The model under review builds one solid part; all positions refer to its coordinate system, in mm. Face numbers are marked on the shaded views. Coordinates: 2 decimals unless noted, no trailing zeros. Loops run counter-clockwise (first coordinate to the right, second up) from the corner with the lowest first, then second, coordinate; pieces in that order, holes last. Notation, with made-up numbers: M 0,64 L 28,64 A34 cw 28,102 Z; hole C -21,32 d11. An arc over 180 degrees is marked long. Use CSV: the item, a comma, the result in double quotes. Start each with the question number.
from build123d import *

# Parameters (mm, degrees)
SKETCH_1_W          = 40
SKETCH_1_H          = 40
EXTRUDE_1_DEPTH     = 60
SKETCH_7_R          = 2.5
CUT_EXTRUDE_1_DEPTH = 10
SKETCH_8_R          = 2.5
CUT_EXTRUDE_2_DEPTH = 10
SKETCH_10_R         = 12.5
CUT_EXTRUDE_3_DEPTH = 40


with BuildPart() as part:
    # 草图1 → 凸台-拉伸1 (new body)
    with BuildSketch(Plane.XY):
        Rectangle(SKETCH_1_W, SKETCH_1_H)
    extrude(amount=EXTRUDE_1_DEPTH)

    # 草图7 → 切除-拉伸1 (cut)
    with BuildSketch(Plane.XZ.offset(20)):
        with Locations(Location((0, 13, 0), (0, 0, 270))):
            Circle(SKETCH_7_R)
    cut_extrude_1 = extrude(amount=-CUT_EXTRUDE_1_DEPTH, mode=Mode.SUBTRACT)

    # 草图8 → 切除-拉伸2 (cut)
    with BuildSketch(Plane(origin=(20, 0, 0), x_dir=(0, 0, -1), z_dir=(1, 0, 0))):
        with Locations((-13, 0)):
            Circle(SKETCH_8_R)
    cut_extrude_2 = extrude(amount=-CUT_EXTRUDE_2_DEPTH, mode=Mode.SUBTRACT)

    # 镜向1: 切除-拉伸1 across plane
    add(cut_extrude_1.mirror(Plane.ZX), mode=Mode.SUBTRACT)

    # 镜向2: 切除-拉伸2 across plane
    add(cut_extrude_2.mirror(Plane(origin=(0, 0, 0), x_dir=(0, 0, 1), z_dir=(1, 0, 0))), mode=Mode.SUBTRACT)

    # 草图10 → 切除-拉伸3 (cut)
    with BuildSketch(Plane.XY.offset(60)):
        Circle(SKETCH_10_R)
    extrude(amount=-CUT_EXTRUDE_3_DEPTH, mode=Mode.SUBTRACT)


solid = part.part
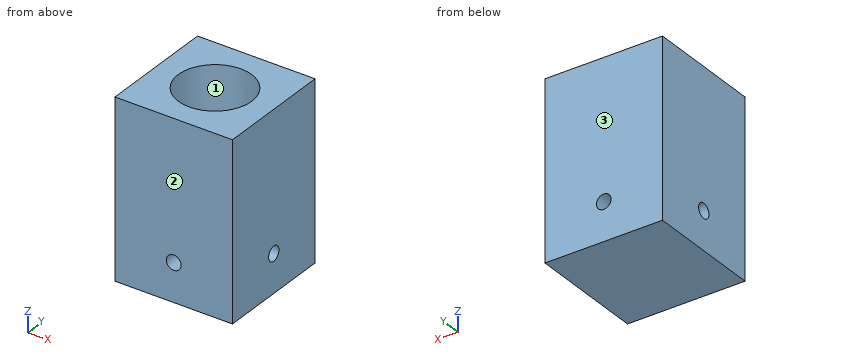
1. Add section B-B (x = 0). Write out the cut boundary in (y, z), plus the area to 3 significant figures.
2. Add section D-D (y = 9). Write out the cut boundary in (x, z), plus the area to 3 significant figures.
3. Add section C-C (z = 28). Write out the cut boundary in (x, y).
4. Add section A-A (z = 11.5). Write out the cut boundary in (x, y), plus the area to 3 significant figures.
5. Insertion check: pin 1 Ø1.5 at (y, z) = (-1, 13.5) entering from +X; pin 2 Ø4.5 at (y, z) = (0, 13) entering from -X. Each pin has a flat end and moves straight along its axis. Give the tip position at first contact, or say it passes through.
6. To check wall thickness, follow line 1 along Y through (x, z) = (-16, 13); line 2 along Y through (x, z) = (0, 40.5). State the ranges of each line that lie inside material, in increasing order.
7. Draft analysis for pull direction Y (two halves, no side actions). For the marked faces 1, 2 and 3, state which applies: released by +Y, released by -Y, zero draft, split by the parting line, or undercut.
Solved:
1,outline,"M -20,0 L 20,0 L 20,10.5 L 10,10.5 L 10,15.5 L 20,15.5 L 20,60 L 12.5,60 L 12.5,20 L -12.5,20 L -12.5,60 L -20,60 L -20,15.5 L -10,15.5 L -10,10.5 L -20,10.5 Z"
1,area,"1,300 mm^2"
2,outline,"M -20,0 L 20,0 L 20,60 L 8.67,60 L 8.67,20 L -8.67,20 L -8.67,60 L -20,60 Z"
2,area,"1,710 mm^2"
3,outline,"M -20,-20 L 20,-20 L 20,20 L -20,20 Z; hole C 0,0 d25"
4,outline,"M -20,-20 L -2,-20 L -2,-10 L 2,-10 L 2,-20 L 20,-20 L 20,-2 L 10,-2 L 10,2 L 20,2 L 20,20 L 2,20 L 2,10 L -2,10 L -2,20 L -20,20 L -20,2 L -10,2 L -10,-2 L -20,-2 Z"
4,area,"1,440 mm^2"
5,pin 1,"stops at x = 10"
5,pin 2,"stops at x = -10"
6,line 1,"y = -20 to -2.5, 2.5 to 20"
6,line 2,"y = -20 to -12.5, 12.5 to 20"
7,face 1,"undercut"
7,face 2,"released by -Y"
7,face 3,"released by +Y"
